Verification items for the finished model (mm, model axes). A direction names the side the tool comes from. Coordinates: 2 decimals unless noted, no trailing zeros. Write each loop counter-clockwise with the first axis right and the second up, starting at its lowest first coordinate (ties: lowest second). Pieces come first, ordered by that corner, then holes. Notation, with made-up numbers: (81, 85.25) -> (90, 85.25) arc R20 ccw to (90, 97.25) -> close; hole circle Ø3 at (6.5, -19). An arc over 180 degrees is marked (long way). Write item = value, one per line. Start each with the question number.
(1) Section check A-A (y = 120.5). Record the cut outline in (x, z).
(2) Mould release check, pull along Y, two halves, no side actions. Record for faces 4 (the face through (58.46, -138.14, 12.32)), 5 (the face through (82.165, -123.621, 12.675)), 6 (the face through (47.69, 15.02, 12.32)), 7 (the face through (-7.025, -118, 12)): released by +Y, released by -Y, zero draft, split by the parting line, or undercut.
(3) Set-up check for faces 1 (the face through (-98.71, -84.57, 12.32)), 2 (the face through (-21.476, -99.021, 12.675)), 3 (the face through (106.182, -48.266, 12.675)): record each of +Z, -Z, +X, -X, +Y, -Y from which the full face is reachable in a straight line by a thin tool's end or side.
(4) Gauge pin test, flat ends, axial feed: pin 1 Ø1.5 at (y, z) = (-42, 4) entering from -X; pin 2 Ø5 at (y, z) = (-21, 3) entering from -X; pin 3 Ø5 at (y, z) = (-87, 21) entering from +X; pin 4 Ø10.5 at (x, y) = (-75.89, -43.82) entering from -Z. Record the tip position at first contact, or that the pin passes through.
(5) Material ranges on probe 1 along Y at (x, z) = (0, 16.25) (3 decimals); probe 2 along X at (y, z) = (-23.5, 20.5); probe 3 along X at (y, z) = (66, 12), recorded low to high. Write a range as [from, to].
(6) Section check B-B (z = 4.75). State how many separate pieces and enclosed holes the cut face has, plus the area to 3 significant figures.
```python
from build123d import *

# Parameters (mm, degrees)
F0_R     = 3
F0_R_2   = 6.605
F0_R_3   = 30
F0_R_4   = 50
F1_DEPTH = 25
F2_R     = 5
F3_R     = 20


with BuildPart() as f1:
    # F0 (on Top) → F1 (new body)
    with BuildSketch(Plane.XY):
        with BuildLine():
            Line((-7.025, -149.835408), (-7.025, -85.932344))
            Line((-7.025, -85.932344), (7.025, -85.932344))
            Line((7.025, -85.932344), (7.025, -114.785232))
            ThreePointArc((7.025, -114.785232), (16.492462, -113.811242), (25.846962, -112.057729))
            Line((25.846962, -112.057729), (30.732203, -146.818022))
            ThreePointArc((30.732203, -146.818022), (58.765568, -138.009449), (84.543744, -123.904622))
            Line((84.543744, -123.904622), (62.870433, -96.292828))
            ThreePointArc((62.870433, -96.292828), (71.005576, -90.461087), (78.602796, -83.944032))
            Line((78.602796, -83.944032), (100.276107, -111.555826))
            ThreePointArc((100.276107, -111.555826), (121.248185, -88.311254), (136.938486, -61.219694))
            Line((136.938486, -61.219694), (104.009355, -49.061736))
            ThreePointArc((104.009355, -49.061736), (107.881617, -39.831604), (110.936591, -30.299716))
            Line((110.936591, -30.299716), (143.865722, -42.457674))
            ThreePointArc((143.865722, -42.457674), (149.325238, 14.211734), (133.273769, 68.833875))
            Line((133.273769, 68.833875), (77.932093, 36.882344))
            Line((77.932093, 36.882344), (70.907093, 49.050001))
            Line((70.907093, 49.050001), (126.248769, 81.001532))
            ThreePointArc((126.248769, 81.001532), (0, 150), (-126.248769, 81.001532))
            Line((-126.248769, 81.001532), (-70.907093, 49.050001))
            Line((-70.907093, 49.050001), (-77.932093, 36.882344))
            Line((-77.932093, 36.882344), (-133.273769, 68.833875))
            ThreePointArc((-133.273769, 68.833875), (-148.903864, -18.100808), (-112.90112, -98.758985))
            Line((-112.90112, -98.758985), (-73.873014, -59.730878))
            ThreePointArc((-73.873014, -59.730878), (-47.5, -82.272413), (-14.791951, -93.841346))
            Line((-14.791951, -93.841346), (-29.077229, -147.154731))
            ThreePointArc((-29.077229, -147.154731), (-18.100808, -148.903864), (-7.025, -149.835408))
        make_face()
        with Locations((-43.815, -75.889806)):
            Circle(F0_R, mode=Mode.SUBTRACT)
        with Locations((-75.889806, -43.815)):
            Circle(F0_R_2, mode=Mode.SUBTRACT)
        with Locations((-85, 0)):
            Circle(F0_R_3, mode=Mode.SUBTRACT)
        Circle(F0_R_4, mode=Mode.SUBTRACT)
        with Locations((75.889806, -43.815)):
            Circle(F0_R_2, mode=Mode.SUBTRACT)
        with Locations((87.63, 0)):
            Circle(F0_R, mode=Mode.SUBTRACT)
        with Locations((-43.815, 75.889806)):
            Circle(F0_R, mode=Mode.SUBTRACT)
        with Locations((42.5, 73.612159)):
            Circle(F0_R_3, mode=Mode.SUBTRACT)
        with Locations((0, 87.63)):
            Circle(F0_R_2, mode=Mode.SUBTRACT)
    extrude(amount=F1_DEPTH)

    # F2
    f2_edges = [f1.edges().sort_by_distance(p)[0] for p in [
        (-77.932093, 36.882344, 12.5),
        (-70.907093, 49.050001, 12.5),
        (70.907093, 49.050001, 12.5),
        (77.932093, 36.882344, 12.5),
        (110.936591, -30.299716, 12.5),
        (104.009355, -49.061736, 12.5),
        (78.602796, -83.944032, 12.5),
        (62.870433, -96.292828, 12.5),
        (25.846962, -112.057729, 12.5),
        (7.025, -114.785232, 12.5),
        (7.025, -85.932344, 12.5),
        (-7.025, -85.932344, 12.5),
        (-7.025, -149.835408, 12.5),
        (-29.077229, -147.154731, 12.5),
        (-112.90112, -98.758985, 12.5),
        (30.732203, -146.818022, 12.5),
        (84.543744, -123.904622, 12.5),
        (100.276107, -111.555826, 12.5),
        (136.938486, -61.219694, 12.5),
        (143.865722, -42.457674, 12.5),
        (133.273769, 68.833875, 12.5),
        (126.248769, 81.001532, 12.5),
        (-126.248769, 81.001532, 12.5),
        (-133.273769, 68.833875, 12.5),
    ]]
    fillet(f2_edges, radius=F2_R)

    # F3
    f3_edges = [f1.edges().sort_by_distance(p)[0] for p in [
        (-73.873014, -59.730878, 12.5),
        (-14.791951, -93.841346, 12.5),
    ]]
    fillet(f3_edges, radius=F3_R)


solid = f1.part
```
Response:
q1.outline = (-89.33, 0) -> (89.33, 0) -> (89.33, 25) -> (-89.33, 25) -> close
q2.face_4 = released by -Y
q2.face_5 = undercut
q2.face_6 = undercut
q2.face_7 = zero draft
q3.face_1 = +Z, -Z, -Y
q3.face_2 = +Z, -Z
q3.face_3 = +Z, -Z, +X
q4.pin_1 = -144.22
q4.pin_2 = -148.85
q4.pin_3 = 123.93
q4.pin_4 = through
q5.probe_1 = [-85.932, -50], [50, 81.025], [94.235, 150]
q5.probe_2 = [-148.15, -103.65], [-66.35, -44.13], [44.13, 148.15]
q5.probe_3 = [-133.92, -128.37], [-100.27, 13.48], [71.52, 100.27], [128.37, 133.92]
q6.separate_pieces = 1
q6.enclosed_holes = 9
q6.area = 47,300 mm2
